Geometry check sheet. Reference: the model listing, model coordinates, mm. Coordinates: 2 decimals unless noted, no trailing zeros. Write each loop counter-clockwise with the first axis right and the second up, starting at its lowest first coordinate (ties: lowest second). Pieces come first, ordered by that corner, then holes. Notation, with made-up numbers: M -34.75,12.5 L -21.75,12.5 A29 cw -21.75,45.5 Z; hole C 12,-22 d11. An arc over 180 degrees is marked long. Put each result on its own line as item: value. Start each with the question number.
1) Cross-section at C-C on x = -71. Record the cut outline in (y, z).
2) Cross-section at A-A on x = 11.5. Record the cut outline in (y, z), plus the area to 3 significant figures.
3) Cross-section at B-B on z = 1.35. Count the separate pieces of the cut face and the enclosed holes in it, plus the area to 3 significant figures.
4) Scan lines: line 1 along Y through (x, z) = (-78.5, 1.3); line 2 along X through (y, z) = (65.5, 0.5); line 3 along Y through (x, z) = (-37, 1.6). Record each from-to range of solid material in increasing order.
5) Gauge pin test, flat ends, axial feed: pin 1 (8 mm diameter, centred on x = -44.5, y = 56.5, fed in from -Z); pin 2 (0.6 mm diameter, centred on x = 46, z = 0.5, fed in from -Y); pin 3 (1 mm diameter, centred on x = 60, z = 1, fed in from +Y); pin 4 (3 mm diameter, centred on x = -78.5, y = -49.5, fed in from -Z). Record the tip position at first contact, or that the pin passes through.
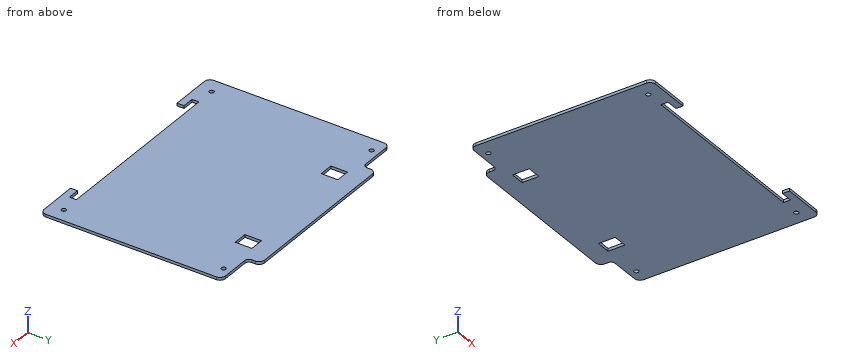
Solid Edge part; units mm, degrees
sketch "Sketch1" plane through (0, 0, 0) normal (0, 0, 1) x (1, 0, 0)
  arc A0 (-64.1, 71) -> (-61.1, 74) centre (-64.1, 74) ccw
  line L0 (-61.1, 74) -> (-61.1, 76.5)
  arc A1 (-61.1, 76.5) -> (-57.1, 80.5) centre (-57.1, 76.5) cw
  line L1 (-57.1, 80.5) -> (0, 80.5)
  line L2 (0, 80.5) -> (57.1, 80.5)
  arc A2 (57.1, 80.5) -> (61.1, 76.5) centre (57.1, 76.5) cw
  line L3 (61.1, 74) -> (61.1, 76.5)
  arc A3 (61.1, 74) -> (64.1, 71) centre (64.1, 74) ccw
  line L4 (78.5, 71) -> (64.1, 71)
  line L5 (78.5, 71) -> (84.5, 71)
  arc A4 (84.5, 71) -> (88.5, 67) centre (84.5, 67) cw
  line L6 (88.5, 67) -> (88.5, -55.5)
  arc A5 (84.5, -59.5) -> (88.5, -55.5) centre (84.5, -55.5) ccw
  line L7 (84.5, -59.5) -> (56.5, -59.5)
  line L8 (56.5, -59.5) -> (56.5, -54.5)
  line L9 (65, -54.5) -> (56.5, -54.5)
  line L10 (65, -49.5) -> (65, -54.5)
  line L11 (-65, -49.5) -> (65, -49.5)
  line L12 (-65, -54.5) -> (-65, -49.5)
  line L13 (-56.5, -54.5) -> (-65, -54.5)
  line L14 (-56.5, -59.5) -> (-56.5, -54.5)
  line L15 (-85.5, -59.5) -> (-56.5, -59.5)
  arc A6 (-89.5, -55.5) -> (-85.5, -59.5) centre (-85.5, -55.5) ccw
  line L16 (-89.5, 8) -> (-89.5, -55.5)
  line L17 (-89.5, 8) -> (-89.5, 67)
  arc A7 (-89.5, 67) -> (-85.5, 71) centre (-85.5, 67) cw
  line L18 (-85.5, 71) -> (-64.1, 71)
  circle A8 centre (78.5, -49.5) radius 1.6
  circle A9 centre (-78.5, -49.5) radius 1.6
  circle A10 centre (-78.5, 65.5) radius 1.6
  line L19 (-50.7, 55) -> (-40.5, 55)
  line L20 (-40.5, 55) -> (-40.5, 67)
  line L21 (-40.5, 67) -> (-50.7, 67)
  line L22 (-50.7, 67) -> (-50.7, 55)
  line L23 (50.7, 55) -> (40.5, 55)
  line L24 (40.5, 55) -> (40.5, 67)
  line L25 (40.5, 67) -> (50.7, 67)
  line L26 (50.7, 67) -> (50.7, 55)
  circle A11 centre (78.5, 65.5) radius 1.6
extrude "Protrusion1" add sketch "Sketch1" along normal blind 2
Answer key:
1. outline: M -59.5,0 L 71,0 L 71,2 L -59.5,2 Z
2. outline: M -49.5,0 L 80.5,0 L 80.5,2 L -49.5,2 Z
2. area: 260 mm²
3. separate pieces: 1
3. enclosed holes: 6
3. area: 22,900 mm²
4. line 1: y = -59.5 to -51.1, -47.9 to 63.9, 67.1 to 71
4. line 2: x = -89.5 to -80.1, -76.9 to -50.7, -40.5 to 40.5, 50.7 to 76.9, 80.1 to 88.5
4. line 3: y = -49.5 to 80.5
5. pin 1: stops at z = 0
5. pin 2: stops at y = -49.5
5. pin 3: stops at y = 79.7
5. pin 4: passes through
